The listing builds one solid part. Answer for the finished solid, in the listing's coordinates (mm). A direction names the side the tool comes from. Coordinates: 2 decimals unless noted, no trailing zeros. Order: outer loops, then holes, each group sorted by start corner. A loop starts at its lowest first (then second) coordinate and runs counter-clockwise, first axis right, second up.
```python
from build123d import *

# Parameters (mm, degrees)
F3_R            = 10
F5_DEPTH        = 1
F5_COPIES_COUNT = 6


# Not quite as in the source:
# - a pattern or mirror of a feature is missing from the dataset's text; its kind, count and spacing are read off the source's solid


with BuildPart() as f2:
    # F1 (on Front) → F2 (revolve)
    with BuildSketch(Plane.XZ):
        Polygon((17.9380366504, 54.5), (17.9380366504, 87.5), (-15.0619633496, 87.5), (-15.0619633496, 54.5), (-1.0619633496, 54.5), (-1.0619633496, 15), (-9, 15), (-9, 6.5), (29, 6.5), (29, 11), (1.9380366504, 11), (1.9380366504, 54.5), align=None)
    revolve(axis=Axis((-1.7091594636, 0, 0), (1, 0, 0)))

    # F3
    f3_edges = [f2.edges().sort_by_distance(p)[0] for p in [
        (17.938037, 0, -54.5),
        (-15.061963, 0, -54.5),
    ]]
    fillet(f3_edges, radius=F3_R)

    # F4 (on Front) → F5 (join, symmetric)
    with BuildSketch(Plane.XZ):
        with BuildLine():
            ThreePointArc((21.256512031, 11.1461849883), (12.8744275284, 33.3890012192), (14.6401561797, 57.0931024849))
            Line((14.6401561797, 57.0931024849), (2.0852813032, 57.0931024849))
            Line((2.0852813032, 57.0931024849), (2.0852813032, 11.0397199169))
            Line((2.0852813032, 11.0397199169), (21.256512031, 11.1461849883))
        make_face()
    f5 = extrude(amount=F5_DEPTH, both=True)

    # F5_copies: F5 ×6 about axis
    f5_copies_axis = Axis((0, 0, 0), (1, 0, 0))
    for i in range(1, F5_COPIES_COUNT):
        add(f5.rotate(f5_copies_axis, i * 360 / F5_COPIES_COUNT))


solid = f2.part
```
(1) Consider line 1 (Y direction, x = -2, z = 0); line 2 (Y direction, x = 6, z = 0). Determine where each line is inside the solid, lowest interval first.
(2) Find section D-D (z = 71). Write down the section's boundary in (x, y).
(3) Find section B-B (x = 5). Write down the section's boundary in (y, z).
(4) Each of these flat-tipped pins is pushed along its axis until it touches: pin 1 Ø10 at (x, y) = (-8.5, -54) entering from +Z; pin 2 Ø4 at (x, y) = (-10.5, 30.5) entering from -Z; pin 3 Ø7 at (y, z) = (-29, -21.5) entering from -X; pin 4 Ø10 at (x, z) = (23, -40) entering from +Y. Where does it stop, or does it pass through?
(5) Find section A-A (z = 0). Write down the section's boundary in (x, y), and give its area (3 significant figures).
(6) The mould has two halves that part along Y. Classify faces 4 (the face through (12.924, 0.014, -33.049)), 5 (the face through (1.21, -59.14, -64.49)), 6 (the face through (29, 5, -5)): released by +Y, released by -Y, zero draft, split by the parting line, or undercut.
(7) Find section C-C (x = 23.5). Write down the section's boundary in (y, z).
(8) For faces 1 (the face through (10.266, 3.955, -5.158)), 2 (the face through (9, -1, -29)), 3 (the face through (-1.062, 11, 11)), determine the directions among +Z, -Z, +X, -X, +Y, -Y from which every point of the face is accessible in a straight line to the end or side of a thin tool.
Findings below:
1. line 1: y = -87.5 to -54.5, -15 to -6.5, 6.5 to 15, 54.5 to 87.5
1. line 2: y = -87.5 to -54.5, -11 to -6.5, 6.5 to 11, 54.5 to 87.5
2. outline: (-15.06, -51.14) - (17.94, -51.14) - (17.94, 51.14) - (-15.06, 51.14) - close
3. outline: circle Ø175 at (0, 0); circle Ø22 at (0, 0); hole (-47.69, -26.38) - (-10.07, -4.66) - (-9.07, -6.39) - (-46.69, -28.11) arc R54.5 ccw to (-1, -54.49) - (-1, -11.06) - (1, -11.06) - (1, -54.49) arc R54.5 ccw to (46.69, -28.11) - (9.07, -6.39) - (10.07, -4.66) - (47.69, -26.38) arc R54.5 ccw to (47.69, 26.38) - (10.07, 4.66) - (9.07, 6.39) - (46.69, 28.11) arc R54.5 ccw to (1, 54.49) - (1, 11.06) - (-1, 11.06) - (-1, 54.49) arc R54.5 ccw to (-46.69, 28.11) - (-9.07, 6.39) - (-10.07, 4.66) - (-47.69, 26.38) arc R54.5 ccw to start; hole circle Ø13 at (0, 0)
4. pin 1: stops at z = 72.49
4. pin 2: stops at z = -82.73
4. pin 3: stops at x = -1.06
4. pin 4: passes through
5. outline: (-15.06, -87.5) - (17.94, -87.5) - (17.94, -64.5) arc R10 ccw to (7.94, -54.5) - (1.94, -54.5) - (1.94, -11) - (29, -11) - (29, -6.5) - (-9, -6.5) - (-9, -15) - (-1.06, -15) - (-1.06, -54.5) - (-5.06, -54.5) arc R10 ccw to (-15.06, -64.5) - close; (-15.06, 64.5) arc R10 ccw to (-5.06, 54.5) - (-1.06, 54.5) - (-1.06, 15) - (-9, 15) - (-9, 6.5) - (29, 6.5) - (29, 11) - (1.94, 11) - (1.94, 54.5) - (7.94, 54.5) arc R10 ccw to (17.94, 64.5) - (17.94, 87.5) - (-15.06, 87.5) - close
5. area: 2,760 mm2
6. face 4: undercut
6. face 5: split by the parting line
6. face 6: zero draft
7. outline: circle Ø22 at (0, 0); hole circle Ø13 at (0, 0)
8. face 1: +X, -X
8. face 2: +X
8. face 3: -X
